The listing builds one solid part. Answer for the finished solid, in the listing's coordinates (mm). Give positions to 0.01 mm unless a question says otherwise; leave off trailing zeros. Loops run counter-clockwise (first coordinate to the right, second up) from the corner with the lowest first, then second, coordinate; pieces in that order, holes last. Notation, with made-up numbers: (17.5, 9.5) - (32.5, 9.5) arc R12 ccw to (32.5, 30.5) - close; hole circle Ø7 at (-36.75, 88.5). An arc over 180 degrees is marked (long way). Write each question's results on one line, items separated by ' | '.
from build123d import *

# Parameters (mm, degrees)
SKETCH1_W             = 12.7
SKETCH1_H             = 3.175
BOSS_EXTRUDE1_DEPTH   = 234.95
F_6_CLEARANCE_HOLE1_D = 3.7973


with BuildPart() as part:
    # Sketch1 → Boss-Extrude1 (new body)
    with BuildSketch(Plane(origin=(0, 0, 0), x_dir=(0, 0, -1), z_dir=(1, 0, 0))):
        Rectangle(SKETCH1_W, SKETCH1_H)
    extrude(amount=-BOSS_EXTRUDE1_DEPTH)

    # #6 Clearance Hole1 (through all)
    with Locations(Plane(origin=(0, 1.5875, 0), x_dir=(1, 0, 0), z_dir=(0, 1, 0))):
        with Locations((-222.25, 0)):
            Hole(F_6_CLEARANCE_HOLE1_D / 2)


solid = part.part
Item 1: Find the intervals of material crossed by line 1 along Z through (x, y) = (-222.25, 0.65); line 2 along X through (y, z) = (1.45, 1.25); line 3 along X through (y, z) = (0.9, -1), in increasing order. Write a range as [from, to].
Values found:
line 1: z = [-6.35, -1.9], [1.9, 6.35] | line 2: x = [-234.95, -223.68], [-220.82, 0] | line 3: x = [-234.95, -223.86], [-220.64, 0]
Item 2: A cutting plane is placed at B-B, the plane z = 0. Determine the outline of the cut face in (x, y), plus the area to 3 significant figures.
Values found:
outline: (-234.95, -1.59) - (-224.15, -1.59) - (-224.15, 1.59) - (-234.95, 1.59) - close; (-220.35, -1.59) - (0, -1.59) - (0, 1.59) - (-220.35, 1.59) - close | area: 734 mm²
Item 3: For a pull along X with two mould halves and no side action, classify faces 1 (the face through (-116, -1.588, 0)), 2 (the face through (-220.353, -0.022, -0.083)) as released by +X, released by -X, zero draft, split by the parting line, or undercut.
Values found:
face 1: zero draft | face 2: undercut
Item 4: A cutting plane is placed at A-A, the plane x = -222.25. Determine the outline of the cut face in (y, z), plus the area to 3 significant figures.
Values found:
outline: (-1.59, -6.35) - (1.59, -6.35) - (1.59, -1.9) - (-1.59, -1.9) - close; (-1.59, 1.9) - (1.59, 1.9) - (1.59, 6.35) - (-1.59, 6.35) - close | area: 28.3 mm²
